Source: three-view drawing plus pictorial views. Frame: mm from the lowest corner of the part. A direction names the side the tool comes from. Give positions to 0.01 mm unless a question says otherwise; leave off trailing zeros. Loops run counter-clockwise (first coordinate to the right, second up) from the corner with the lowest first, then second, coordinate; pieces in that order, holes last. Notation, with made-up numbers: (28.5, 8) - (48.5, 8) arc R25 ccw to (48.5, 47) - close; hole circle Ø3 at (-18, -35.5). An arc over 180 degrees is marked (long way). Put each result on its own line as item: value.
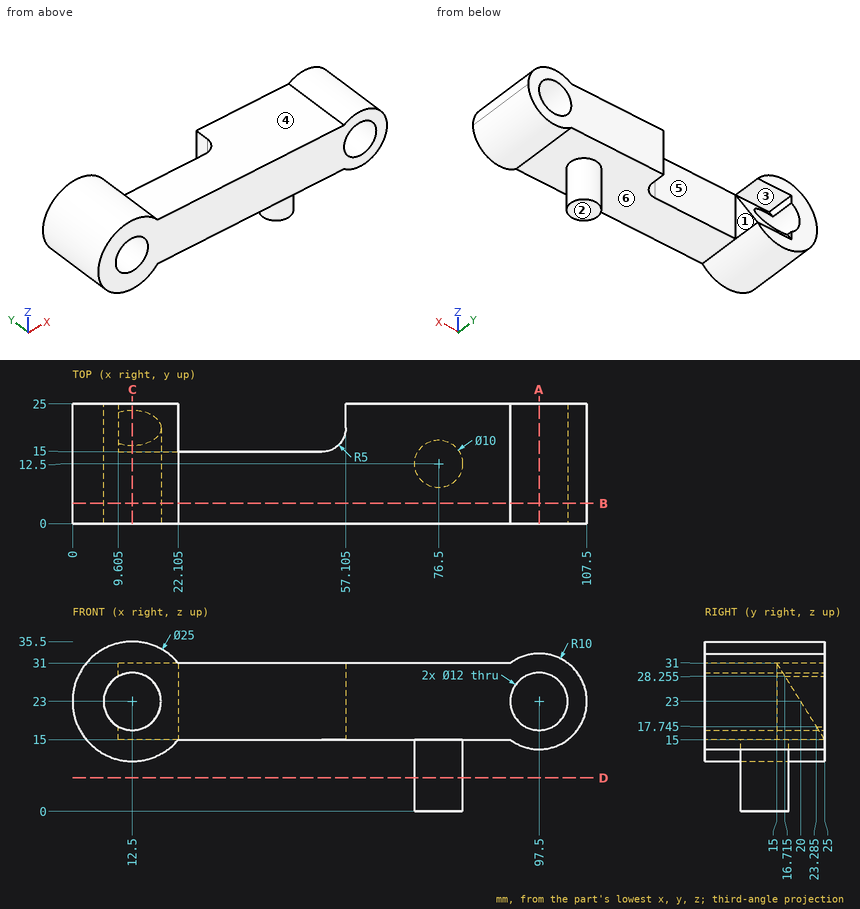
1) Section query D-D, the plane z = 7. Output: boundary loops of the cut face in (x, y).
Check result:
outline: circle Ø10 at (76.5, 12.5)
2) Section query C-C, the plane x = 12.5. Output: boundary loops of the cut face in (y, z).
Check result:
outline: (0, 10.5) - (25, 10.5) - (25, 15) - (23.75, 17) - (0, 17) - close; (0, 29) - (16.25, 29) - (15, 31) - (25, 31) - (25, 35.5) - (0, 35.5) - close
3) Access query for the marked faces 4, 5 and 6. Directions: +Z, -Z, +X, -X, +Y, -Y. A direction counts if a zero-diameter tool reaches every point of the face in a straight line with its end or side. Return the directions, or none.
Check result:
face 4: +Z, +Y, -Y
face 5: +Z, -Z, +Y
face 6: -Z
4) Material intervals for line 1 along Z through (x, y) = (97.5, 19.75); line 2 along Z through (x, y) = (12.5, 18.75); line 3 along Z through (x, y) = (41.5, 8.5), sorted ascending. Write a range as [from, to].
Check result:
line 1: [13, 17], [29, 33]
line 2: [10.5, 17], [31, 35.5]
line 3: [15, 31]
5) Mould query, pull axis Z, two halves, no side actions, for the marked faces 1, 2 and 3. Classes: pulls with the +Z half, pulls with the -Z half, needs draft (parallel to the pull), parting line crosses it, or undercut.
Check result:
face 1: needs draft
face 2: pulls with the -Z half
face 3: undercut
6) Section query A-A, the plane x = 97.5. Output: boundary loops of the cut face in (y, z).
Check result:
outline: (0, 13) - (25, 13) - (25, 17) - (0, 17) - close; (0, 29) - (25, 29) - (25, 33) - (0, 33) - close
7) Pin query (flat end, axial travel): P1, Ø8, axis at y = 16.5, z = 28, coming from the -X side; P2, Ø6, axis at y = 4.5, z = 9.5, coming from the -X side (1 decimal); P3, Ø12.5, axis at x = 46.5, y = 9.5, coming from the -Z side; P4, Ø7, axis at x = 12.5, z = 23, coming from the +Y side. Return the tip coordinate at first contact, or that it passes through.
Check result:
P1: x = 0.04
P2: x = 5.7
P3: z = 15
P4: through
8) Section query B-B, the plane y = 4.25. Output: boundary loops of the cut face in (x, z) (1 decimal), plus the area to 3 significant figures.
Check result:
outline: (22.1, 15) - (91.5, 15) arc R10 ccw (long way) to (91.5, 31) - (22.1, 31) arc R12.5 ccw (long way) to start; hole circle Ø12 at (12.5, 23); hole circle Ø12 at (97.5, 23)
area: 1,610 mm²
